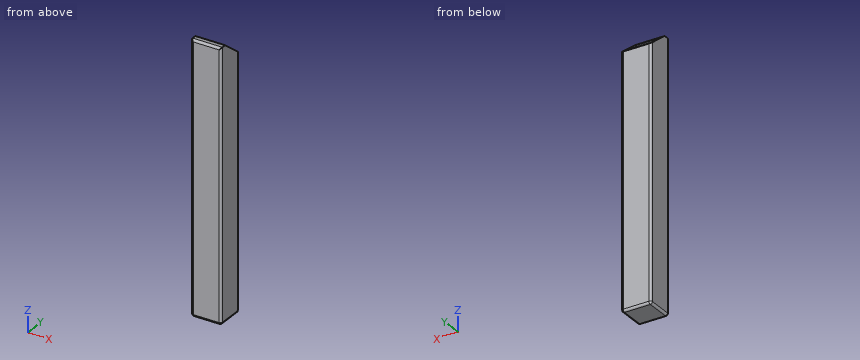
from build123d import *

# Parameters (mm, degrees)
SKETCH1_W           = 177.8
SKETCH1_H           = 1587.5
BOSS_EXTRUDE1_DEPTH = 165.1
CUT_EXTRUDE1_DEPTH  = 177.8
SHELL2_T            = -6.35
FILLET3_R           = 12.7


with BuildPart() as part:
    # Sketch1 → Boss-Extrude1 (new body)
    with BuildSketch(Plane(origin=(0, 0, 0), x_dir=(1, 0, 0), z_dir=(0, 1, 0))):
        with Locations((88.9, 793.75)):
            Rectangle(SKETCH1_W, SKETCH1_H)
    extrude(amount=BOSS_EXTRUDE1_DEPTH)

    # Sketch2 → Cut-Extrude1 (cut)
    with BuildSketch(Plane(origin=(177.8, 0, 0), x_dir=(0, 0, -1), z_dir=(1, 0, 0))):
        Polygon((0, 165.1), (98.317886998, 165.1), (0, 38.1), align=None)
    extrude(amount=-CUT_EXTRUDE1_DEPTH, mode=Mode.SUBTRACT)

    # Shell2
    shell2_openings = [part.faces().sort_by_distance(p)[0] for p in [
        (88.9, 101.6, -49.158943499),
    ]]
    offset(amount=SHELL2_T, openings=shell2_openings, kind=Kind.INTERSECTION)

    # Fillet3
    fillet3_edges = [part.edges().sort_by_distance(p)[0] for p in [
        (177.8, 165.1, -842.908943499),
        (88.9, 165.1, -1587.5),
        (0, 165.1, -842.908943499),
        (88.9, 0, -1587.5),
        (177.8, 0, -793.75),
        (88.9, 0, 0),
        (0, 0, -793.75),
        (0, 82.55, -1587.5),
        (177.8, 82.55, -1587.5),
    ]]
    fillet(fillet3_edges, radius=FILLET3_R)


solid = part.part
Design review of the part built by this model. Coordinates are the model's own, in mm. Round coordinates to 2 decimals unless told otherwise and drop trailing zeros. Write each loop counter-clockwise with the first axis right and the second up, starting at its lowest first coordinate (ties: lowest second). Pieces come first, ordered by that corner, then holes. Notation, with made-up numbers: (3, 35) -> (12, 35) arc R31 cw to (12, 60) -> close; hole circle Ø5 at (-36.75, 26). An arc over 180 degrees is marked (long way). One line per question, with ' | ' between items.
(1) Take a section at A-A, the plane z = -1214. State the section outline as (x, y) points, and give its area (3 significant figures).
Result sheet:
outline: (0, 12.7) arc R12.7 ccw to (12.7, 0) -> (165.1, 0) arc R12.7 ccw to (177.8, 12.7) -> (177.8, 152.4) arc R12.7 ccw to (165.1, 165.1) -> (12.7, 165.1) arc R12.7 ccw to (0, 152.4) -> close; hole (6.35, 6.35) -> (171.45, 6.35) -> (171.45, 158.75) -> (6.35, 158.75) -> close | area: 4,060 mm2
(2) Insertion check: P1, Ø1.5, axis at x = 21, y = 53.5, coming from the +Z side. The pin has a flat end and moves straight along its axis. Give the tip position at first contact, or say it passes through.
Result sheet:
P1: z = -1581.15
(3) Wall thickness on line 1 (Y direction, x = 39.5, z = -789); line 2 (X direction, y = 34.5, z = -617); line 3 (Z direction, x = 69, y = 12): over which ranges is each line inside the solid? List them lowest first. Write a range as [from, to].
Result sheet:
line 1: [0, 6.35], [158.75, 165.1] | line 2: [0, 6.35], [171.45, 177.8] | line 3: [-1587.48, -1581.15], [-6.35, -0.02]
(4) Take a section at C-C, the plane y = 114.5. State the section outline as (x, z) points.
Result sheet:
outline: (0, -1574.8) arc R12.7 ccw to (12.7, -1587.5) -> (165.1, -1587.5) arc R12.7 ccw to (177.8, -1574.8) -> (177.8, -59.15) -> (171.45, -59.15) -> (171.45, -1581.15) -> (6.35, -1581.15) -> (6.35, -59.15) -> (0, -59.15) -> close
(5) Take a section at B-B, the plane x = 130. State the section outline as (y, z) points, and give its area (3 significant figures).
Result sheet:
outline: (0, -1574.8) arc R12.7 ccw to (12.7, -1587.5) -> (152.4, -1587.5) arc R12.7 ccw to (165.1, -1574.8) -> (165.1, -98.32) -> (158.75, -93.4) -> (158.75, -1581.15) -> (6.35, -1581.15) -> (6.35, -6.35) -> (46.3, -6.35) -> (38.1, 0) -> (12.7, 0) arc R12.7 ccw to (0, -12.7) -> close | area: 20,600 mm2
